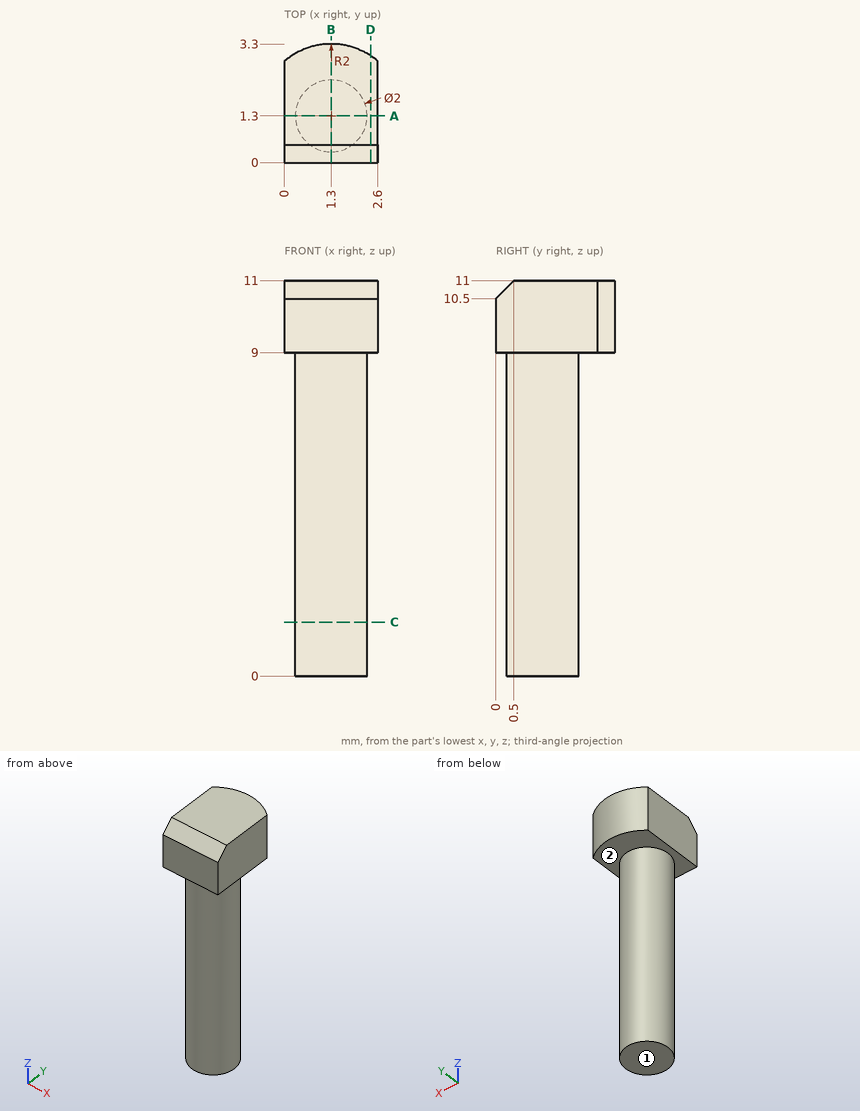
Study the drawing (mm; zero at the part's minimum x, y, z) and answer. A direction names the side the tool comes from. Round coordinates to 2 decimals unless told otherwise and drop trailing zeros. Write each loop counter-clockwise with the first axis right and the second up, starting at its lowest first coordinate (ties: lowest second). Pieces come first, ordered by that corner, then holes.
1) Which of the six approach directions +Z, -Z, +X, -X, +Y, -Y give full straight-line access (tool end or side, diameter ignored) to the marked faces 1 and 2?
2) A cutting plane is placed at A-A on y = 1.3. Determine the outline of the cut face in (x, z).
3) A flat-ended cylindrical pin translates along its axis: P1, Ø1, axis at y = 2.5, z = 3, coming from the -X side. Find the tip coordinate at first contact, or state that the pin passes through.
4) Consider probe 1 along Z at (x, y) = (2.15, 1.9); probe 2 along Y at (x, z) = (1.3, 3.25). Determine where each line is inside the solid, lowest interval first.
5) A cutting plane is placed at B-B on x = 1.3. Determine the outline of the cut face in (y, z), and give its area (3 significant figures).
6) A cutting plane is placed at D-D on x = 2.4. Determine the outline of the cut face in (y, z), and give its area (3 significant figures).
7) A cutting plane is placed at C-C on z = 1.5. Determine the outline of the cut face in (x, y).
Entries:
1. face 1: -Z, +X, -X, +Y, -Y
1. face 2: -Z
2. outline: (0, 9) - (0.3, 9) - (0.3, 0) - (2.3, 0) - (2.3, 9) - (2.6, 9) - (2.6, 11) - (0, 11) - close
3. P1: stops at x = 0.59
4. probe 1: z = 9 to 11
4. probe 2: y = 0.3 to 2.3
5. outline: (0, 9) - (0.3, 9) - (0.3, 0) - (2.3, 0) - (2.3, 9) - (3.3, 9) - (3.3, 11) - (0.5, 11) - (0, 10.5) - close
5. area: 24.5 mm2
6. outline: (0, 9) - (2.97, 9) - (2.97, 11) - (0.5, 11) - (0, 10.5) - close
6. area: 5.82 mm2
7. outline: circle Ø2 at (1.3, 1.3)
